```python
from build123d import *

# Parameters (mm, degrees)
F0_W     = 30
F0_H     = 18
F1_DEPTH = 5
F2_R     = 2.25
F3_DEPTH = 5
F5_START = -2
F5_DEPTH = 7
F7_DEPTH = 7
F8_W     = 5
F8_H     = 12
F9_DEPTH = 18


with BuildPart() as f1:
    # F0 (on Top) → F1 (new body)
    with BuildSketch(Plane.XY):
        Rectangle(F0_W, F0_H)
    extrude(amount=F1_DEPTH)

    # F2 (on face) → F3 (cut, through all)
    with BuildSketch(Plane.XY.offset(5)):
        with Locations((-5, 5.5)):
            Circle(F2_R)
        with Locations((-5, -5.5)):
            Circle(F2_R)
    extrude(amount=-F3_DEPTH, mode=Mode.SUBTRACT)

    # F4 (on face) → F5 (join)
    with BuildSketch(Plane.XZ.offset(9).offset(F5_START)):
        with BuildLine():
            Line((15, 5), (15, 10))
            ThreePointArc((15, 10), (9.9983587547, 14.9999997306), (5.0000010775, 9.9967175095))
            Line((5.0000010775, 9.9967175095), (5.0000010775, 5))
            Line((5.0000010775, 5), (15, 5))
        make_face()
    extrude(amount=-F5_DEPTH)

    # F6 (on face) → F7 (cut, through all)
    with BuildSketch(Plane.XZ.offset(7)):
        with BuildLine():
            Line((7.7483587547, 9.9967175095), (12.2483587547, 9.9967175095))
            ThreePointArc((12.2483587547, 9.9967175095), (9.9983587547, 12.2467175095), (7.7483587547, 9.9967175095))
        make_face()
        with BuildLine():
            ThreePointArc((7.7483587547, 9.9967175095), (9.9983587547, 7.7467175095), (12.2483587547, 9.9967175095))
            Line((12.2483587547, 9.9967175095), (7.7483587547, 9.9967175095))
        make_face()
    extrude(amount=-F7_DEPTH, mode=Mode.SUBTRACT)

    # F8 (on face) → F9 (join)
    with BuildSketch(Plane.XZ.offset(9)):
        with Locations((-12.5, 11)):
            Rectangle(F8_W, F8_H)
    extrude(amount=-F9_DEPTH)


solid = f1.part
```
Design review of the part built by this model. Coordinates are the model's own, in mm. A direction names the side the tool comes from. Give positions to 0.01 mm unless a question says otherwise; leave off trailing zeros. Order: outer loops, then holes, each group sorted by start corner. A loop starts at its lowest first (then second) coordinate and runs counter-clockwise, first axis right, second up. Notation, with made-up numbers: (-12, 62) - (7, 62) arc R16 ccw to (7, 86) - close; hole circle Ø10 at (13.5, 7.25). An arc over 180 degrees is marked (long way). Use a Markdown table: item, result. Add a question column.
(1) Add section A-A on y = 5.5. Give the boundary of the cut face in (x, z).
(2) Add section C-C on x = -5. Give the boundary of the cut face in (y, z).
(3) Add section D-D on x = 9. Give the boundary of the cut face in (y, z), then the cut area to 3 significant figures.
(4) Wall thickness on probe 1 along Y at (x, z) = (-5, 1.2); probe 2 along X at (y, z) = (7.75, 6.5); probe 3 along Y at (x, z) = (6.75, 12.5): over which ranges is each line inside the solid? List them lowest first. Write a range as [from, to].
(5) Machinability: for faces 1 (the face through (11, -7, 7.8)), 2 (the face through (-10, 0, 11)), 3 (the face through (-15, 0, 8)), which of the approach directions +Z, -Z, +X, -X, +Y, -Y give a long, thin tool a straight path to every point of the face, cutting with its end or side? Answer none if there is none.
(6) Mouldability with a two-part tool opening along X and no side actions: class faces 4 (the face through (2, 0, 5)), 5 (the face through (11, 0, 7.8)), 6 (the face through (15, 0, 4)), 7 (the face through (10, -4, 15)) as +X half, -X half, draft (parallel to the pull), parting line (faces both ways), or undercut.
(7) Clearance check with flat-ended pins moving along their axes: P1, Ø4, axis at x = 5.5, y = 7, coming from the +Z side; P2, Ø3, axis at x = 8.5, z = 7.5, coming from the -Y side; P3, Ø4, axis at x = -5, y = -5.5, coming from the +Z side; P4, Ø1, axis at x = 8.5, y = 0, coming from the +Z side. State where each tip first meets the part, or that it passes through.
(8) Add section B-B on y = -5.5. Give the boundary of the cut face in (x, z).
Report:
| question | item | result |
|---|---|---|
| 1 | outline | (-15, 0) - (-7.25, 0) - (-7.25, 5) - (-10, 5) - (-10, 17) - (-15, 17) - close; (-2.75, 0) - (15, 0) - (15, 5) - (-2.75, 5) - close |
| 2 | outline | (-9, 0) - (-7.75, 0) - (-7.75, 5) - (-9, 5) - close; (-3.25, 0) - (3.25, 0) - (3.25, 5) - (-3.25, 5) - close; (7.75, 0) - (9, 0) - (9, 5) - (7.75, 5) - close |
| 3 | outline | (-9, 0) - (9, 0) - (9, 5) - (0, 5) - (0, 7.98) - (-7, 7.98) - (-7, 5) - (-9, 5) - close; (-7, 12.01) - (0, 12.01) - (0, 14.9) - (-7, 14.9) - close |
| 3 | area | 131 mm² |
| 4 | probe 1 | y = [-9, -7.75], [-3.25, 3.25], [7.75, 9] |
| 4 | probe 2 | x = [-15, -10] |
| 4 | probe 3 | y = [-7, 0] |
| 5 | face 1 | +Z, +X, -Y |
| 5 | face 2 | +Z, +Y, -Y |
| 5 | face 3 | +Z, -Z, -X, +Y, -Y |
| 6 | face 4 | undercut |
| 6 | face 5 | draft |
| 6 | face 6 | +X half |
| 6 | face 7 | undercut |
| 7 | P1 | stops at z = 5 |
| 7 | P2 | stops at y = -7 |
| 7 | P3 | passes through |
| 7 | P4 | stops at z = 14.9 |
| 8 | outline | (-15, 0) - (-7.25, 0) - (-7.25, 5) - (-10, 5) - (-10, 17) - (-15, 17) - close; (-2.75, 0) - (15, 0) - (15, 10) arc R5 ccw to (5, 10) - (5, 5) - (-2.75, 5) - close; hole circle Ø4.5 at (10, 10) |
